```python
from build123d import *

# Parameters (mm, degrees)
BOSS_EXTRUDE1_DEPTH              = 6.35
SKETCH2_W                        = 19.05
SKETCH2_H                        = 44.45
CUT_EXTRUDE1_DEPTH               = 199.119607398
F_17_64_0_26563_DIAMETER_HOLE1_D = 6.747002
F_1_4_CLEARANCE_HOLE1_D          = 7.14248
SKETCH7_W                        = 3.175
SKETCH7_H                        = 184.33652634
SKETCH7_H_2                      = 154.225553014
CUT_EXTRUDE2_DEPTH               = 199.119607398
FILLET1_R                        = 2.54


with BuildPart() as part:
    # Sketch1 → Boss-Extrude1 (new body)
    with BuildSketch(Plane(origin=(0, 0, 0), x_dir=(1, 0, 0), z_dir=(0, 1, 0))):
        Polygon((0, -76.835), (0, 76.835), (-175.26, 92.16826317), (-175.26, -92.16826317), align=None)
    extrude(amount=BOSS_EXTRUDE1_DEPTH)

    # Sketch2 → Cut-Extrude1 (cut, through all)
    with BuildSketch(Plane(origin=(0, 6.35, 0), x_dir=(1, 0, 0), z_dir=(0, 1, 0))):
        with Locations((-87.63, 84.501631585)):
            Rectangle(SKETCH2_W, SKETCH2_H)
    extrude(amount=-CUT_EXTRUDE1_DEPTH, mode=Mode.SUBTRACT)

    # 17/64 (0.26563) Diameter Hole1 (through all)
    with Locations(Plane(origin=(0, 6.35, 0), x_dir=(1, 0, 0), z_dir=(0, 1, 0))):
        with Locations((-24.485, -42.27), (-64.0721, -42.27), (-111.1879, -42.27), (-150.775, -42.27), (-78.4321, 45.355), (-10.125, 45.355), (-96.8279, 45.355), (-165.135, 45.355)):
            Hole(F_17_64_0_26563_DIAMETER_HOLE1_D / 2)

    # 1/4 Clearance Hole1 (through all)
    with Locations(Plane(origin=(0, 6.35, 0), x_dir=(1, 0, 0), z_dir=(0, 1, 0))):
        with Locations((-25.4, 71.400370648), (-25.4, -71.400370648), (-149.86, -82.28920971), (-151.13, 82.042)):
            Hole(F_1_4_CLEARANCE_HOLE1_D / 2)

    # Sketch7 → Cut-Extrude2 (cut, through all)
    with BuildSketch(Plane(origin=(0, 6.35, 0), x_dir=(1, 0, 0), z_dir=(0, 1, 0))):
        with Locations((-173.6725, 0)):
            Rectangle(SKETCH7_W, SKETCH7_H)
        with Locations((-1.5875, 0)):
            Rectangle(SKETCH7_W, SKETCH7_H_2)
    extrude(amount=-CUT_EXTRUDE2_DEPTH, mode=Mode.SUBTRACT)

    # Fillet1
    fillet1_edges = [part.edges().sort_by_distance(p)[0] for p in [
        (-172.085, 3.175, -91.890486663),
        (-172.085, 3.175, 91.890486663),
        (-3.175, 3.175, 77.112776507),
        (-3.175, 3.175, -77.112776507),
        (-97.155, 3.175, -85.334961105),
        (-97.155, 3.175, -62.276631585),
        (-78.105, 3.175, -83.668302065),
        (-78.105, 3.175, -62.276631585),
    ]]
    fillet(fillet1_edges, radius=FILLET1_R)


solid = part.part
```
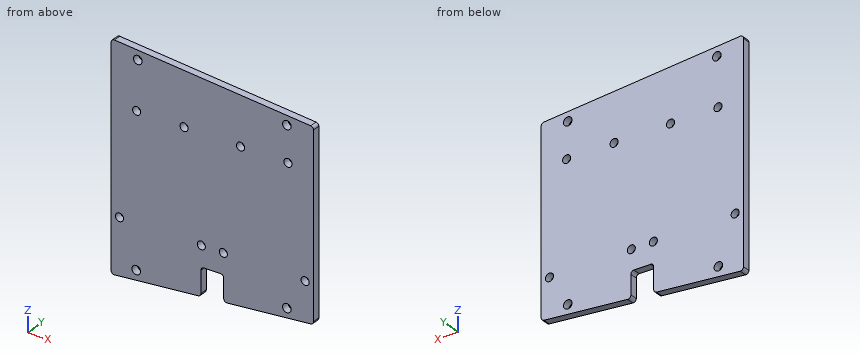
Work out the finished part from the listing and answer in its coordinate system (mm). Give positions to 0.01 mm unless a question says otherwise; leave off trailing zeros. Order: outer loops, then holes, each group sorted by start corner. A loop starts at its lowest first (then second) coordinate and runs counter-clockwise, first axis right, second up. Notation, with made-up numbers: (-9.5, -26) - (-2.5, -26) arc R22 cw to (-2.5, -17) - close; hole circle Ø3 at (29, 87). An arc over 180 degrees is marked (long way). One line per item, written item: value. Start each with the question number.
1. Section B-B, the plane x = -149.86 is taken. Write down the section's boundary in (y, z), then the cut area to 3 significant figures.
2. Section A-A, the plane z = 42.27 is taken. Count the separate pieces of the cut face and the enclosed holes in it, then the cut area to 3 significant figures.
3. Each of these flat-tipped pins is pushed along its axis until it touches: pin 1 Ø8 at (x, z) = (-25.4, 71.4) entering from -Y; pin 2 Ø1 at (x, y) = (-21, 4) entering from +Z. Where does it stop, or does it pass through?
4. Section D-D, the plane x = -25 is taken. Write down the section's boundary in (y, z), then the cut area to 3 significant figures.
5. Consider line 1 (X direction, y = 1.5, z = 42.27) (1 decimal); line 2 (Z direction, x = -149.86, y = 2); line 3 (Z direction, x = -111, y = 5). Determine where each line is inside the solid, lowest interval first.
Filled sheet:
1. outline: (0, -89.95) - (6.35, -89.95) - (6.35, -85.38) - (0, -85.38) - close; (0, -78.7) - (6.35, -78.7) - (6.35, 39.02) - (0, 39.02) - close; (0, 45.52) - (6.35, 45.52) - (6.35, 78.72) - (0, 78.72) - close; (0, 85.86) - (6.35, 85.86) - (6.35, 89.95) - (0, 89.95) - close
1. area: 1,010 mm²
2. separate pieces: 5
2. enclosed holes: 0
2. area: 901 mm²
3. pin 1: y = 0
3. pin 2: z = 78.72
4. outline: (0, -79.02) - (6.35, -79.02) - (6.35, -74.95) - (0, -74.95) - close; (0, -67.85) - (6.35, -67.85) - (6.35, 38.94) - (0, 38.94) - close; (0, 45.6) - (6.35, 45.6) - (6.35, 67.85) - (0, 67.85) - close; (0, 74.95) - (6.35, 74.95) - (6.35, 79.02) - (0, 79.02) - close
4. area: 871 mm²
5. line 1: -172.1 to -154.1, -147.4 to -114.6, -107.8 to -67.4, -60.7 to -27.9, -21.1 to -3.2
5. line 2: -89.95 to -85.38, -78.7 to 39.02, 45.52 to 78.72, 85.86 to 89.95
5. line 3: -86.55 to 38.9, 45.64 to 86.55
